```python
from build123d import *


with BuildPart() as part:
    # Sweep1: sweep along a path in Sketch1
    with BuildLine(Plane.XY) as sweep1_path:
        Line((-2.798998946, 12.182594342), (51.286022129, 24.608840571))
        ThreePointArc((51.286022129, 24.608840571), (82.19, 0), (51.286022129, -24.608840571))
        Line((51.286022129, -24.608840571), (-2.798998946, -12.182594342))
        ThreePointArc((-2.798998946, -12.182594342), (-12.5, 0), (-2.798998946, 12.182594342))
    # Sketch2 → Sweep1 (sweep)
    with BuildSketch(Plane(origin=(-2.798998946, 0, 0), x_dir=(0, 0, -1), z_dir=(1, 0, 0))):
        Polygon((0, 12.21966763), (-3, 12.21966763), (-3, 13.21966763), (3, 13.21966763), (3, 12.21966763), align=None)
    sweep(path=sweep1_path.line)


solid = part.part
```
Here's how the part is built. I have some questions about the finished solid (model axes, mm). A direction names the side the tool comes from. Coordinates: 2 decimals unless noted, no trailing zeros. Loops run counter-clockwise (first coordinate to the right, second up) from the corner with the lowest first, then second, coordinate; pieces in that order, holes last. Notation, with made-up numbers: M -25,40 L 32,40 A17 ccw 32,73 Z; hole C -20.75,3 d4. An arc over 180 degrees is marked long. One line per item, written item: value.
1. Imagine slicing it at C-C (y = 0). List the corners of the cut face in (x, z) for me, and give its area (3 significant figures).
Geometry says:
outline: M -13.51,-3 L -12.54,-3 L -12.54,3 L -13.51,3 Z; M 82.23,-3 L 83.2,-3 L 83.2,3 L 82.23,3 Z
area: 11.7 mm2
2. Thinking about a two-plate mould opening in Y: for faces 3 (the cylindrical face through (83.2, 0.4, 0)), 4 (the flat face through (23.41, -19.24, -0.04)), 5 (the flat face through (23.849, -18.342, 0.042)), 6 (the cylindrical face through (-12.534, -0.228, -0.042)), which applies, +Y half, -Y half, draft (parallel to the pull), parting line (faces both ways), or undercut?
Geometry says:
face 3: parting line
face 4: -Y half
face 5: undercut
face 6: undercut
3. Imagine slicing it at B-B (z = -1.75). List the corners of the cut face in (x, y) for me.
Geometry says:
outline: M -3.25,-13.12 L 50.83,-25.54 A26.26 ccw long 51.29,25.65 L -2.8,13.22 A13.51 ccw Z; hole M -2.82,-12.22 L 51.27,-24.64 A25.29 ccw long 51.29,24.65 L -2.8,12.22 A12.54 ccw Z
4. Please list where these lines run through material, in increasing order: probe 1 along X at (y, z) = (0, -1.4); probe 2 along Y at (x, z) = (56.94, 1.5); probe 3 along Y at (x, z) = (33.5, -0.75).
Geometry says:
probe 1: x = -13.51 to -12.54, 82.23 to 83.2
probe 2: y = -26.26 to -25.29, 25.29 to 26.26
probe 3: y = -21.56 to -20.56, 20.56 to 21.56
5. On a 3-axis mill with a long thin cutter (end or side, diameter ignored), from which of +Z, -Z, +X, -X, +Y, -Y can I reach the whole of each face in a straight line? I mean faces 1 (the cylindrical face through (-13.513, -0.022, 0.042)), 2 (the flat face through (24.62, 18.52, 0.04)). Say none if no direction works.
Geometry says:
face 1: +Z, -Z, -X
face 2: +Z, -Z
6. Will these pins go through, and if not, where does the flat tip stop? pin 1 Ø2 at (x, z) = (4.5, 0) entering from -Y; pin 2 Ø2 at (x, z) = (58.5, 0.5) entering from +Y; pin 3 Ø1 at (y, z) = (-17.5, -2.5) entering from +X.
Geometry says:
pin 1: stops at y = -15.13
pin 2: stops at y = 26.26
pin 3: stops at x = 76.96
7. Imagine slicing it at A-A (x = 56.94). List the corners of the cut face in (y, z) for me.
Geometry says:
outline: M -26.26,-3 L -25.29,-3 L -25.29,3 L -26.26,3 Z; M 25.29,-3 L 26.26,-3 L 26.26,3 L 25.29,3 Z
